Geometry: final body of the model. Coordinates: model frame, mm. A direction names the side the tool comes from. Give positions to 0.01 mm unless a question says otherwise; leave off trailing zeros. Order: outer loops, then holes, each group sorted by start corner. A loop starts at its lowest first (then second) coordinate and runs counter-clockwise, first axis right, second up. Notation, with made-up numbers: (-11, 26) -> (5, 26) arc R29 ccw to (5, 46) -> close; hole circle Ø5 at (70, 85). An arc over 180 degrees is marked (long way). Answer in a Markdown table with one row per item. Add a question column.
Q1. Cut plane B-B on x = -9. Return the cut outline in (y, z), and give its area (3 significant figures).
Q2. Cut plane C-C on y = -9.5. Return the cut outline in (x, z).
Q3. Set-up query: faces 1 (the face through (0, 0, 10.5)), 2 (the face through (6.586, 10.329, 4.754)), 3 (the face through (0, 0, 4)). Return all of +Z, -Z, +X, -X, +Y, -Y with unobstructed straight access to the full face (end or side cutting, diameter ignored); none if empty.
Q4. Cut plane A-A on y = 0. Return the cut outline in (x, z), and give its area (4 significant figures).
Q5. Contact query for flat-ended pins moving along their axis: P1, Ø1, axis at y = -12.5, z = 4.5, coming from the -X side; P2, Ø4, axis at x = 4.5, z = 2.5, coming from the +Y side; P3, Ø5, axis at y = -8.5, z = 6.5, coming from the +X side; P4, Ø5.5, axis at x = 7.25, y = 0, coming from the -Z side. Output: stop coordinate, or through.
Q6. Pull-direction query (Y, two-part tool) for faces 4 (the face through (4, -12, 5)), 5 (the face through (0.391, -4.276, 4.246)), 6 (the face through (7.123, 11.172, 3.124)), 7 (the face through (0, -3, 4.5)); classes: +Y half, -Y half, draft (parallel to the pull), parting line (faces both ways), or undercut.
Q7. Cut plane D-D on z = 2.75. Return the cut outline in (x, y).
Q8. Line query: line 1 along Y through (x, z) = (0, 4.25); line 2 along Y through (x, z) = (2.5, 4.25); line 3 along Z through (x, y) = (-13, 2). Output: solid intervals per line, ascending. Write a range as from..to.
from build123d import *

# Parameters (mm, degrees)
SKETCH1_R           = 17.75
BOSS_EXTRUDE1_DEPTH = 1.3
SKETCH2_R           = 13.25
BOSS_EXTRUDE2_DEPTH = 3.7
SKETCH3_R           = 12
CUT_EXTRUDE1_DEPTH  = 4
SKETCH4_R           = 12.25
CUT_EXTRUDE2_DEPTH  = 0.5
SKETCH5_R           = 3
CUT_EXTRUDE3_DEPTH  = 0.5
SKETCH6_R           = 1.15
BOSS_EXTRUDE3_DEPTH = 6


with BuildPart() as part:
    # Sketch1 → Boss-Extrude1 (new body)
    with BuildSketch(Plane.XY):
        Circle(SKETCH1_R)
    extrude(amount=BOSS_EXTRUDE1_DEPTH)

    # Sketch2 → Boss-Extrude2 (add)
    with BuildSketch(Plane.XY.offset(1.3)):
        Circle(SKETCH2_R)
    extrude(amount=BOSS_EXTRUDE2_DEPTH)

    # Sketch3 → Cut-Extrude1 (cut)
    with BuildSketch(Plane(origin=(0, 0, 0), x_dir=(-1, 0, 0), z_dir=(0, 0, -1))):
        Circle(SKETCH3_R)
    extrude(amount=-CUT_EXTRUDE1_DEPTH, mode=Mode.SUBTRACT)

    # Sketch4 → Cut-Extrude2 (cut)
    with BuildSketch(Plane.XY.offset(5)):
        Circle(SKETCH4_R)
    extrude(amount=-CUT_EXTRUDE2_DEPTH, mode=Mode.SUBTRACT)

    # Sketch5 → Cut-Extrude3 (cut)
    with BuildSketch(Plane(origin=(0, 0, 4), x_dir=(-1, 0, 0), z_dir=(0, 0, -1))):
        with Locations((0, 7.25)):
            Circle(SKETCH5_R)
        with Locations((7.25, 0)):
            Circle(SKETCH5_R)
        with Locations((0, -7.25)):
            Circle(SKETCH5_R)
        with Locations((-7.25, 0)):
            Circle(SKETCH5_R)
    extrude(amount=-CUT_EXTRUDE3_DEPTH, mode=Mode.SUBTRACT)

    # Sketch6 → Boss-Extrude3 (add)
    with BuildSketch(Plane.XY.offset(4.5)):
        Circle(SKETCH6_R)
    extrude(amount=BOSS_EXTRUDE3_DEPTH)


solid = part.part
Completed:
| question | item | result |
|---|---|---|
| 1 | outline | (-15.3, 0) -> (-7.94, 0) -> (-7.94, 4) -> (-2.44, 4) -> (-2.44, 4.5) -> (-8.31, 4.5) -> (-8.31, 5) -> (-9.72, 5) -> (-9.72, 1.3) -> (-15.3, 1.3) -> close; (2.44, 4) -> (7.94, 4) -> (7.94, 0) -> (15.3, 0) -> (15.3, 1.3) -> (9.72, 1.3) -> (9.72, 5) -> (8.31, 5) -> (8.31, 4.5) -> (2.44, 4.5) -> close |
| 1 | area | 37.5 mm² |
| 2 | outline | (-14.99, 0) -> (-7.33, 0) -> (-7.33, 4) -> (-1.98, 4) -> (-1.98, 4.5) -> (-7.73, 4.5) -> (-7.73, 5) -> (-9.24, 5) -> (-9.24, 1.3) -> (-14.99, 1.3) -> close; (1.98, 4) -> (7.33, 4) -> (7.33, 0) -> (14.99, 0) -> (14.99, 1.3) -> (9.24, 1.3) -> (9.24, 5) -> (7.73, 5) -> (7.73, 4.5) -> (1.98, 4.5) -> close |
| 3 | face 1 | +Z, +X, -X, +Y, -Y |
| 3 | face 2 | +Z |
| 3 | face 3 | -Z |
| 4 | outline | (-17.75, 0) -> (-12, 0) -> (-12, 4) -> (-10.25, 4) -> (-10.25, 4.5) -> (-12.25, 4.5) -> (-12.25, 5) -> (-13.25, 5) -> (-13.25, 1.3) -> (-17.75, 1.3) -> close; (-4.25, 4) -> (4.25, 4) -> (4.25, 4.5) -> (1.15, 4.5) -> (1.15, 10.5) -> (-1.15, 10.5) -> (-1.15, 4.5) -> (-4.25, 4.5) -> close; (10.25, 4) -> (12, 4) -> (12, 0) -> (17.75, 0) -> (17.75, 1.3) -> (13.25, 1.3) -> (13.25, 5) -> (12.25, 5) -> (12.25, 4.5) -> (10.25, 4.5) -> close |
| 4 | area | 43.75 mm² |
| 5 | P1 | stops at x = -5.62 |
| 5 | P2 | stops at y = 17.51 |
| 5 | P3 | stops at x = 11.55 |
| 5 | P4 | passes through |
| 6 | face 4 | draft |
| 6 | face 5 | undercut |
| 6 | face 6 | parting line |
| 6 | face 7 | undercut |
| 7 | outline | circle Ø26.5 at (0, 0); hole circle Ø24 at (0, 0) |
| 8 | line 1 | y = -13.25..-10.25, -4.25..4.25, 10.25..13.25 |
| 8 | line 2 | y = -13.01..-8.91, -5.59..5.59, 8.91..13.01 |
| 8 | line 3 | z = 0..5 |
